Input: part model. Units: mm. Frame: model coordinates. A direction names the side the tool comes from. Round coordinates to 2 decimals unless told otherwise and drop trailing zeros. Loops run counter-clockwise (first coordinate to the right, second up) from the corner with the lowest first, then second, coordinate; pieces in that order, holes last. Notation, with made-up numbers: (69, 86) - (119, 86) arc R6 cw to (119, 93) - close; hole circle Ø5 at (25, 46.25). An arc over 180 degrees is marked (long way). One line per question, with ' | ' between items. Start each with the question number.
Item 1: Draft query along Y for faces 5 (the face through (-44.55, -0.18, 4.57)), 6 (the face through (-9.47, 2.95, 10.76)), 7 (the face through (-5, 7.5, 10)). Return one class per face: pulls with the +Y half, pulls with the -Y half, needs draft (parallel to the pull), parting line crosses it, or undercut.
Item 2: Material intervals for line 1 along X through (y, z) = (5, 2.3); line 2 along Y through (x, z) = (37.5, 3.25); line 3 along Z through (x, y) = (-4.7, 0), sorted ascending.
Item 3: Set-up query: faces 1 (the face through (-9.472, -3.814, 14.743)), 2 (the face through (-7.5, -3.2, 16.3)), 3 (the face through (-11.5, 0.4, 8.9)), 4 (the face through (-9, 0, 8.075)). Return all of +Z, -Z, +X, -X, +Y, -Y with unobstructed straight access to the full face (end or side cutting, diameter ignored); none if empty.
Item 4: Section A-A, the plane x = 37.5. Return loops of the section in (y, z), plus the area to 3 significant figures.
Item 5: Section C-C, the plane x = -21.5. Return loops of the section in (y, z).
Item 6: Section B-B, the plane y = -11.5. Return loops of the section in (x, z).
Item 7: First-contact query: pin 1 (1.2 mm diameter, centred on x = -9.5, y = 0, fed in from +Z) (3 decimals); pin 2 (6.5 mm diameter, centred on y = 3, z = 15, fed in from +X); pin 3 (5.5 mm diameter, centred on y = -1, z = 13.5, fed in from -X). Flat tips, straight axial feed; report the tip coordinate or a pass-through.
Autodesk Fusion 360 part; units mm, degrees
sketch "Sketch1" plane through (0, 0, 0) normal (0, 0, 1) x (1, 0, 0)
  line L0 (-45, 14) -> (45, 14)
  line L1 (45, 14) -> (45, -14)
  line L2 (45, -14) -> (-45, -14)
  line L3 (-45, -14) -> (-45, 14)
  line L4 (-45, 14) -> (45, -14) construction
  line L5 (45, 14) -> (-45, -14) construction
  dimension "d1" = 90
  dimension "d2" = 28
extrude "Extrude1" add sketch "Sketch1" along normal blind 5
sketch "Sketch2" plane through (0, 0, 0) normal (0, 0, 1) x (1, 0, 0)
  line L0 (0, 0) -> (37.5, 0)
  line L1 (0, 0) -> (-37.5, 0)
  circle A0 centre (37.5, 0) radius 2
  circle A1 centre (-37.5, 0) radius 2
  dimension "d5" = 37.5
  dimension "d6" = 37.5
  dimension "d7" = 4
  dimension "d8" = 4
sketch "Sketch3" plane through (0, 0, 0) normal (0, 0, 1) x (1, 0, 0)
  line L0 (0, 0) -> (-37.5, 0)
  circle A0 centre (-37.5, 0) radius 2
  dimension "d11" = 37.5
  dimension "d12" = 4
ref_plane "WorkPlane1" through (0, 0, 5) normal (0, 0, 1) x (1, 0, 0)
sketch "Sketch4" plane through (0, 0, 5) normal (0, 0, 1) x (1, 0, 0)
  line L0 (0, 0) -> (-5, 0)
  line L1 (-2.5, 7.5) -> (-7.5, 7.5)
  line L2 (-7.5, 7.5) -> (-7.5, -7.5)
  line L3 (-7.5, -7.5) -> (-2.5, -7.5)
  line L4 (-2.5, -7.5) -> (-2.5, 7.5)
  line L5 (-2.5, 7.5) -> (-7.5, -7.5) construction
  line L6 (-7.5, 7.5) -> (-2.5, -7.5) construction
  point P0 (-5, 0)
  dimension "d16" = 5
  dimension "d17" = 5
  dimension "d18" = 15
extrude "Extrude4" add sketch "Sketch4" along normal blind 15
sketch "Sketch5" plane through (0, 0, 5) normal (0, 0, 1) x (-1, 0, 0)
  line L0 (2.5, 7.5) -> (7.5, 7.5)
  line L1 (7.5, 7.5) -> (7.5, -7.5)
  line L2 (7.5, -7.5) -> (2.5, -7.5)
  line L3 (2.5, -7.5) -> (2.5, 7.5)
  line L4 (45, 14) -> (-45, 14)
  line L5 (-45, 14) -> (-45, -14)
  line L6 (-45, -14) -> (45, -14)
  line L7 (45, -14) -> (45, 14)
  line L8 (0, 0) -> (-5, 0)
  line L9 (-7.5, -7.5) -> (-2.5, -7.5)
  line L10 (-2.5, -7.5) -> (-2.5, 7.5)
  line L11 (-2.5, 7.5) -> (-7.5, 7.5)
  line L12 (-7.5, 7.5) -> (-7.5, -7.5)
  line L13 (-7.5, -7.5) -> (-2.5, 7.5) construction
  line L14 (-2.5, -7.5) -> (-7.5, 7.5) construction
  point P0 (-5, 0)
  dimension "d23" = 5
  dimension "d24" = 5
  dimension "d25" = 15
hole "Hole1" at (7.5, 0, 9.3622) direction (-1, 0, 0) diameter 4.5 depth 6 tip angle 118
hole "Hole2" at (-2.5, 0, 12.5) direction (-1, 0, 0) diameter 4.5 depth 6 tip angle 118
fillet "Fillet3" radius 1.5 2 edges at (0, 14, 5) (0, -14, 5)
sketch "Sketch6" plane through (0, 0, 0) normal (0, 0, 1) x (1, 0, 0)
  line L0 (0, 0) -> (37.5, 0)
  line L1 (37.5, 0) -> (37.5, 5)
  line L2 (0, 0) -> (-37.5, 0)
  line L3 (-37.5, 0) -> (-37.5, 5)
  dimension "d38" = 37.5
  dimension "d39" = 5
  dimension "d40" = 37.5
  dimension "d41" = 5
hole "Hole3" at (-37.5, 5, 0) direction (0, 0, 1) diameter 4.5 depth 5 tip angle 118
sketch "Sketch7" plane through (0, 0, 0) normal (0, 0, 1) x (1, 0, 0)
  line L0 (0, 0) -> (37.5, 0)
  line L1 (37.5, 0) -> (37.5, 5)
  dimension "d45" = 37.5
  dimension "d46" = 5
hole "Hole4" at (37.5, 5, 0) direction (0, 0, 1) diameter 4.5 depth 5 tip angle 118
fillet "Fillet4" radius 1.5 10 edges at (-45, 14, 1.75) (-45, 13.5607, 4.5607) (-45, 0, 5) (-45, -13.5607, 4.5607) (-45, -14, 1.75) (45, -14, 1.75) (45, -13.5607, 4.5607) (45, 0, 5) (45, 13.5607, 4.5607) (45, 14, 1.75)
fillet "Fillet5" radius 7.5 2 edges at (-5, -7.5, 20) (-5, 7.5, 20)
fillet "Fillet6" radius 2 4 edges at (-5, -7.5, 5) (-2.5, 0, 5) (-5, 7.5, 5) (-7.5, 0, 5)
sketch "Sketch8" plane through (-2.5, 0, 0) normal (1, 0, 0) x (0, 1, 0)
  line L0 (-7.5, 7) -> (7.5, 7)
  line L1 (7.5, 7) -> (7.5, 12.5)
  arc A0 (7.5, 12.5) -> (-7.5, 12.5) centre (0, 12.5) ccw
  line L2 (-7.5, 12.5) -> (-7.5, 7)
  circle A1 centre (0, 12.5) radius 2.25
  line L3 (1.9774, 15.925) -> (-1.9774, 15.925)
  line L4 (-1.9774, 15.925) -> (-3.9548, 12.5)
  line L5 (-3.9548, 12.5) -> (-1.9774, 9.075)
  line L6 (-1.9774, 9.075) -> (1.9774, 9.075)
  line L7 (1.9774, 9.075) -> (3.9548, 12.5)
  line L8 (3.9548, 12.5) -> (1.9774, 15.925)
  line L9 (-5.1095, 12.5) -> (-2.5548, 8.075)
  line L10 (-2.5548, 8.075) -> (2.5548, 8.075)
  line L11 (2.5548, 8.075) -> (5.1095, 12.5)
  line L12 (5.1095, 12.5) -> (2.5548, 16.925)
  line L13 (2.5548, 16.925) -> (-2.5548, 16.925)
  line L14 (-2.5548, 16.925) -> (-5.1095, 12.5)
  point P0 (0, 12.5)
  dimension "d56" = 6.85
  dimension "d57" = 1
extrude "Extrude6" add sketch "Sketch8" against normal blind 4 from surface at -5 contours L9 L10 L11 L12 L13 L14
Return value:
1) face 5: needs draft | face 6: undercut | face 7: pulls with the +Y half
2) line 1: -45 to -39.75, -35.25 to 35.25, 39.75 to 45 | line 2: -14 to 2.75, 7.25 to 14 | line 3: 0 to 10.25, 14.75 to 20
3) face 1: +Z, -X, -Y | face 2: -X | face 3: +Z, -X, +Y, -Y | face 4: -X, +Y, -Y
4) outline: (-14, 0) - (2.75, 0) - (2.75, 5) - (-12.5, 5) arc R1.5 ccw to (-14, 3.5) - close; (7.25, 0) - (14, 0) - (14, 3.5) arc R1.5 ccw to (12.5, 5) - (7.25, 5) - close | area: 117 mm2
5) outline: (-14, 0) - (14, 0) - (14, 3.5) arc R1.5 ccw to (12.5, 5) - (-12.5, 5) arc R1.5 ccw to (-14, 3.5) - close
6) outline: (-45, 0) - (45, 0) - (45, 3.5) arc R1.5 ccw to (43.5, 5) - (-43.5, 5) arc R1.5 ccw to (-45, 3.5) - close
7) pin 1: z = 16.925 | pin 2: x = -2.5 | pin 3: x = -11.5
